Model file for the job. Use its own axes, mm. A direction names the side the tool comes from. Coordinates: 2 decimals unless noted, no trailing zeros. Loops run counter-clockwise (first coordinate to the right, second up) from the corner with the lowest first, then second, coordinate; pieces in that order, holes last. Notation, with made-up numbers: (49.5, -37) -> (56.5, -37) arc R21 cw to (56.5, -9) -> close; hole circle Ø2 at (8, -22.5). An arc over 180 degrees is marked (long way). Use one line per item in the form item = value.
```python
from build123d import *

# Parameters (mm, degrees)
F0_W     = 50.8
F0_H     = 25.4
F1_DEPTH = 11.43
F2_R     = 2.54
F3_R     = 2.54
F4_R     = 0.508
F5_DEPTH = 6.096
F6_DEPTH = 0.0508


with BuildPart() as f1:
    # F0 (on Top) → F1 (new body)
    with BuildSketch(Plane.XY):
        Rectangle(F0_W, F0_H)
    extrude(amount=F1_DEPTH)

    # F2
    f2_edges = [f1.edges().sort_by_distance(p)[0] for p in [
        (25.4, -12.7, 5.715),
        (-25.4, -12.7, 5.715),
        (25.4, 12.7, 5.715),
        (-25.4, 12.7, 5.715),
    ]]
    fillet(f2_edges, radius=F2_R)

    # F3
    f3_edges = [f1.edges().sort_by_distance(p)[0] for p in [
        (0, 12.7, 11.43),
    ]]
    fillet(f3_edges, radius=F3_R)

    # F4 (on face) → F5 (join)
    with BuildSketch(Plane(origin=(0, 0, 0), x_dir=(1, 0, 0), z_dir=(0, 0, -1))):
        with Locations((22.86, 7.62)):
            Circle(F4_R)
        with Locations((22.86, -2.54)):
            Circle(F4_R)
        with Locations((22.86, -7.62)):
            Circle(F4_R)
        with Locations((-22.86, -10.16)):
            Circle(F4_R)
        with Locations((-22.86, 0)):
            Circle(F4_R)
        with Locations((-22.86, 10.16)):
            Circle(F4_R)
    extrude(amount=F5_DEPTH)

    # F4 (on face) → F6 (join)
    with BuildSketch(Plane(origin=(0, 0, 0), x_dir=(1, 0, 0), z_dir=(0, 0, -1))):
        with Locations((-22.86, -10.16)):
            Circle(F4_R)
        with Locations((-22.86, 0)):
            Circle(F4_R)
        with Locations((-22.86, 10.16)):
            Circle(F4_R)
        with Locations((22.86, 7.62)):
            Circle(F4_R)
        with Locations((22.86, -2.54)):
            Circle(F4_R)
        with Locations((22.86, -7.62)):
            Circle(F4_R)
        with Locations((-20.32, -10.16)):
            Circle(F4_R)
        with Locations((-20.32, 10.16)):
            Circle(F4_R)
        with Locations((20.32, -7.62)):
            Circle(F4_R)
        with Locations((20.32, 7.62)):
            Circle(F4_R)
    extrude(amount=F6_DEPTH)


solid = f1.part
```
Q1. Which spindle directions (+Z, -Z, +X, -X, +Y, -Y) get a long thin tool onto all of the face, cutting with end or side? Do faces 1 (the face through (24.636, -0.142, 10.706)), 2 (the face through (-20, -10, -0.051)), 3 (the face through (20.3, 7.6, -0.051)), 4 (the face through (-22.375, -10.313, -3.005)). Say none if no direction does.
Result:
face_1 = +Z, +X, +Y, -Y
face_2 = -Z, +X, +Y, -Y
face_3 = -Z, -X, +Y, -Y
face_4 = -Z
Q2. Pin check, flat tips, straight feed: pin 1 Ø1.1 at (x, y) = (-20.5, -10) entering from -Z; pin 2 Ø7.5 at (x, y) = (-9.5, -3.5) entering from -Z. Stop position of each tip, or through.
Result:
pin_1 = -0.05
pin_2 = 0
Q3. Band-saw the part on B-B, the plane y = -8.75. Write the cut outline in (x, z).
Result:
outline = (-25.4, 0) -> (25.4, 0) -> (25.4, 8.89) arc R2.54 ccw to (22.86, 11.43) -> (-22.86, 11.43) arc R2.54 ccw to (-25.4, 8.89) -> close
Q4. Wall check: line 1 along Z through (x, y) = (20, -4); line 2 along Y through (x, z) = (22.5, -1); line 3 along X through (y, z) = (-10.25, 8). Give the ranges that are in metal, low to high.
Result:
line_1 = 0 to 11.43
line_2 = -7.98 to -7.26, 2.18 to 2.9, 7.26 to 7.98
line_3 = -25.4 to 25.4
Q5. Band-saw the part on C-C, the plane z = -2.5. Write the cut outline in (x, y), and give its area (3 significant figures).
Result:
outline = circle Ø1.02 at (-22.86, -10.16); circle Ø1.02 at (-22.86, 0); circle Ø1.02 at (-22.86, 10.16); circle Ø1.02 at (22.86, -7.62); circle Ø1.02 at (22.86, 2.54); circle Ø1.02 at (22.86, 7.62)
area = 4.86 mm2
Q6. Band-saw the part on A-A, the plane x = 4. Write the cut outline in (y, z).
Result:
outline = (-12.7, 0) -> (12.7, 0) -> (12.7, 8.89) arc R2.54 ccw to (10.16, 11.43) -> (-10.16, 11.43) arc R2.54 ccw to (-12.7, 8.89) -> close
Q7. Band-saw the part on D-D, the plane x = -20.32. Write the cut outline in (y, z), and give its area (3 significant figures).
Result:
outline = (-12.7, 0) -> (-10.67, 0) -> (-10.67, -0.05) -> (-9.65, -0.05) -> (-9.65, 0) -> (9.65, 0) -> (9.65, -0.05) -> (10.67, -0.05) -> (10.67, 0) -> (12.7, 0) -> (12.7, 8.89) arc R2.54 ccw to (10.16, 11.43) -> (-10.16, 11.43) arc R2.54 ccw to (-12.7, 8.89) -> close
area = 288 mm2
